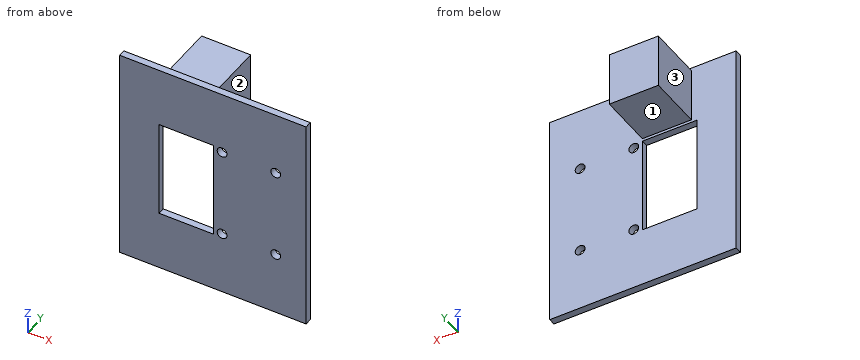
Autodesk Inventor part; units mm, degrees
ref_plane "Work Plane2" through (0, 1.6, 0) normal (0, 1, 0) x (1, 0, 0)
ref_plane "Work Plane1" through (0, 1.6, 0) normal (0, 1, 0) x (1, 0, 0)
ref_plane "YZ Plane" through (0, 0, 0) normal (1, 0, 0) x (0, 1, 0)
sketch "Sketch1" plane through (0, 0, 0) normal (0, 1, 0) x (-1, 0, 0)
  line L0 (21.717, 25.4) -> (-21.717, 25.4)
  line L1 (-21.717, 25.4) -> (-21.717, -25.4)
  line L2 (-21.717, -25.4) -> (21.717, -25.4)
  line L3 (21.717, -25.4) -> (21.717, -11.43)
  line L4 (12.573, -11.43) -> (-0.127, -11.43)
  line L5 (-0.127, -11.43) -> (-0.127, 11.43)
  line L6 (-0.127, 11.43) -> (12.573, 11.43)
  line L7 (21.717, 11.43) -> (21.717, 25.4)
  line L8 (12.573, -11.43) -> (12.573, 11.43)
  line L9 (21.717, 11.43) -> (21.717, -11.43)
  point P0 (0, 0)
  dimension "d0" = 43.434
  dimension "d1" = 43.434
  dimension "d2" = 21.717
  dimension "d3" = 50.8
  dimension "d4" = 25.4
  dimension "d33" = 21.59
  dimension "d34" = 12.7
  dimension "d35" = 13.97
  dimension "d36" = 13.97
ref_plane "Work Plane2" through (0, 1.6, 0) normal (0, 1, 0) x (1, 0, 0)
extrude "Extrusion4" add sketch "Sketch1" along normal blind 1.6
ref_plane "Work Plane1" through (0, 1.6, 0) normal (0, 1, 0) x (1, 0, 0)
sketch "Sketch3" plane through (0, 1.6, 0) normal (0, 1, 0) x (1, 0, 0)
  circle A0 centre (2.1387, -10.5016) radius 1.143
  circle A1 centre (2.1387, 10.5016) radius 1.143
  circle A2 centre (14.638, -10.5016) radius 1.143
  circle A3 centre (14.638, 10.5016) radius 1.143
  line L0 (21.717, -25.4) -> (21.717, 25.4)
  point P0 (0, 0)
  dimension "d19" = 2.286
  dimension "d20" = 2.286
  dimension "d21" = 2.286
  dimension "d22" = 2.286
  dimension "d23" = 21.0033
  dimension "d24" = 21.0033
  dimension "d27" = 12.4993
  dimension "d30" = 12.4993
  dimension "d42" = 7.079
  dimension "d43" = 7.079
  dimension "d44" = 10.5016
extrude "Extrusion6" cut sketch "Sketch3" against normal through all
sketch "Sketch4" plane through (0, 1.6, 0) normal (0, 1, 0) x (1, 0, 0)
  line L0 (-11.303, -24.765) -> (0.127, -24.765)
  line L1 (0.127, -24.765) -> (0.127, -12.065)
  line L2 (0.127, -12.065) -> (-11.303, -12.065)
  line L3 (-11.303, -12.065) -> (-11.303, -24.765)
  line L4 (-12.573, -11.43) -> (-12.573, 11.43)
  line L5 (0.127, 11.43) -> (0.127, -11.43)
  line L6 (-21.717, -25.4) -> (21.717, -25.4)
  point P0 (0, 0)
  dimension "d48" = 0
  dimension "d49" = 11.43
  dimension "d50" = 12.7
  dimension "d51" = 0.635
extrude "Extrusion7" add sketch "Sketch4" along normal blind 12.7
equation "\"d1\" = d0"
equation "\"d36\" = d35"
equation "\"d20\" = d19"
equation "\"d21\" = d20"
equation "\"d22\" = d21"
equation "\"d24\" = d23"
equation "\"d30\" = d27"
equation "\"d43\" = d42"
properties part number "Sensor Board"
Can you work these out from the model? Positions are in its coordinate system, mm. Face numbers are marked on the shaded views. A direction names the side the tool comes from. Round coordinates to 2 decimals unless told otherwise and drop trailing zeros. Loops run counter-clockwise (first coordinate to the right, second up) from the corner with the lowest first, then second, coordinate; pieces in that order, holes last. Notation, with made-up numbers: (46.5, 58) -> (82.5, 58) arc R19 cw to (82.5, 70) -> close; hole circle Ø9 at (83, 86). An arc over 180 degrees is marked (long way). One line per item, written item: value. Start each with the question number.
1. If we section it at A-A, the plane x = -7: Write out the boundary of the cut face in (y, z) (3 decimals).
2. For pin 1 (3.5 mm diameter, centred on x = 2.14, z = -10.5, fed in from +Y); pin 2 (6 mm diameter, centred on x = -8, y = 10.5, fed in from -Z) (3 decimals); pin 3 (6.5 mm diameter, centred on y = 8.5, z = 20, fed in from +X), each with a flat end and sliding along its axis, tell me the tip position at first contact or that it passes through.
3. If we section it at B-B, the plane z = 8: Write out the boundary of the cut face in (x, y), then the cut area to 3 significant figures.
4. If I drill on probe 1 along X at (y, z) = (1.5, 11.5); probe 2 along Y at (x, z) = (14, -15.5); probe 3 along Z at (x, y) = (-1, 6) (3 decimals), over which ranges is the centre line in solid material (lowest first)?
5. For the marked faces 1, 2 and 3, which set-ups out of +Z, -Z, +X, -X, +Y, -Y let a thin tool reach every point of the face, with its end or its side?
6. If we section it at D-D, the plane x = 7: Write out the boundary of the cut face in (y, z), then the cut area to 3 significant figures.
7. If we section it at C-C, the plane y = 4.75: Write out the boundary of the cut face in (x, z) (3 decimals).
Calculated:
1. outline: (0, -25.4) -> (1.6, -25.4) -> (1.6, -11.43) -> (0, -11.43) -> close; (0, 11.43) -> (1.6, 11.43) -> (1.6, 12.065) -> (14.3, 12.065) -> (14.3, 24.765) -> (1.6, 24.765) -> (1.6, 25.4) -> (0, 25.4) -> close
2. pin 1: stops at y = 1.6
2. pin 2: stops at z = 12.065
2. pin 3: stops at x = 0.13
3. outline: (-21.72, 0) -> (-12.57, 0) -> (-12.57, 1.6) -> (-21.72, 1.6) -> close; (0.13, 0) -> (21.72, 0) -> (21.72, 1.6) -> (0.13, 1.6) -> close
3. area: 49.2 mm²
4. probe 1: x = -21.72 to 1.58, 2.7 to 14.08, 15.19 to 21.72
4. probe 2: y = 0 to 1.6
4. probe 3: z = 12.065 to 24.765
5. face 1: -Z, +X, -X, +Y
5. face 2: +Z, -Z, +X, +Y
5. face 3: +Z, -Z, -X, +Y
6. outline: (0, -25.4) -> (1.6, -25.4) -> (1.6, 25.4) -> (0, 25.4) -> close
6. area: 81.3 mm²
7. outline: (-11.303, 12.065) -> (0.127, 12.065) -> (0.127, 24.765) -> (-11.303, 24.765) -> close
